Check sheet for the modelled part. Datum: model origin and axes. Units: mm. Face numbers are marked on the shaded views. A direction names the side the tool comes from. Round coordinates to 2 decimals unless told otherwise and drop trailing zeros. Loops run counter-clockwise (first coordinate to the right, second up) from the corner with the lowest first, then second, coordinate; pieces in that order, holes last. Notation, with made-up numbers: (-4, 64.25) -> (42, 64.25) arc R30 ccw to (42, 102.25) -> close; hole circle Ø5 at (-21, 32). An arc over 180 degrees is marked (long way). Use one line per item in the form item = value. Start each with the question number.
(1) Sectioned sample at C-C (y = -53). Record the cut outline in (x, z), and give its area (3 significant figures).
(2) Go/stop test with flat-tipped pins: pin 1 (2.5 mm diameter, centred on x = -0.5, y = -47.5, fed in from +Z); pin 2 (1.5 mm diameter, centred on x = 8.5, y = -50.5, fed in from -Z); pin 3 (3 mm diameter, centred on x = 11.5, y = -16.5, fed in from +Z). Record where each tip stops, or that it passes through.
(3) Material ranges on probe 1 along Y at (x, z) = (7.5, 16.25); probe 2 along X at (y, z) = (-26.5, 21); probe 3 along Y at (x, z) = (21, 14), recorded low to high. Write a range as [from, to].
(4) Sectioned sample at B-B (y = -32.5). Record the cut outline in (x, z).
(5) Draft check along X on the marked faces 5, 6, 7 and 8. Enter one of: released by +X, released by -X, zero draft, split by the parting line, or undercut.
(6) Set-up check for the marked faces 1, 2, 3 and 4: record each of +Z, -Z, +X, -X, +Y, -Y from which the full face is reachable in a straight line by a thin tool's end or side.
(7) Sectioned sample at A-A (z = 18). Record the cut outline in (x, y).
(8) Sectioned sample at D-D (z = 4.5). State how many separate pieces and enclosed holes the cut face has, and give its area (3 significant figures).
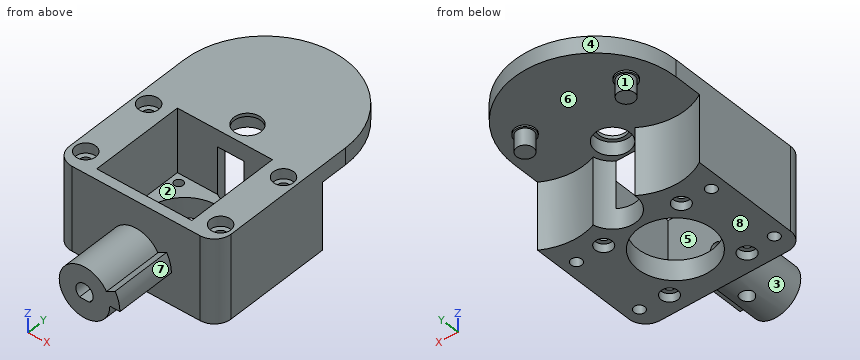
from build123d import *

# Parameters (mm, degrees)
EXTRUDE_1_DEPTH      = 25
SKETCH_3_W           = 28.2
SKETCH_3_H           = 28.2
CUT_EXTRUDE_1_DEPTH  = 19
SKETCH_4_R           = 11.1
CUT_EXTRUDE_2_DEPTH  = 26
CUT_EXTRUDE_3_DEPTH  = 20
SKETCH_11_R          = 3
EXTRUDE_2_DEPTH      = 0.5
SKETCH_12_R          = 2.5
EXTRUDE_3_DEPTH      = 5
SKETCH_13_R          = 5.05
CUT_EXTRUDE_6_DEPTH  = 4
SKETCH_14_R          = 4
CUT_EXTRUDE_7_DEPTH  = 2
SKETCH_15_R          = 1.6
CUT_EXTRUDE_8_DEPTH  = 26
SKETCH_16_R          = 3
CUT_EXTRUDE_9_DEPTH  = 3
SKETCH_17_R          = 1.3
CUT_EXTRUDE_10_DEPTH = 7
SKETCH_18_R          = 2.5
CUT_EXTRUDE_11_DEPTH = 2.5
FILLET_1_R           = 5
SKETCH_19_R          = 7.5
EXTRUDE_4_DEPTH      = 18
CUT_EXTRUDE_12_DEPTH = 18
SKETCH_21_R          = 1.5
CUT_EXTRUDE_13_DEPTH = 10
EXTRUDE_5_DEPTH      = 18
SKETCH_23_R          = 2
CUT_EXTRUDE_14_DEPTH = 8.4


with BuildPart() as part:
    # 草图1 → 凸台-拉伸1 (new body)
    with BuildSketch(Plane.XY):
        with BuildLine():
            Line((-24, 0), (-24, -45))
            Line((-24, -45), (24, -45))
            Line((24, -45), (24, 0))
            ThreePointArc((24, 0), (0, 24), (-24, 0))
        make_face()
    extrude(amount=EXTRUDE_1_DEPTH)

    # 草图3 → 切除-拉伸1 (cut)
    with BuildSketch(Plane.XY.offset(25)):
        with Locations((0, -28)):
            Rectangle(SKETCH_3_W, SKETCH_3_H)
    extrude(amount=-CUT_EXTRUDE_1_DEPTH, mode=Mode.SUBTRACT)

    # 草图4 → 切除-拉伸2 (cut, through all)
    with BuildSketch(Plane(origin=(0, 0, 0), x_dir=(-1, 0, 0), z_dir=(0, 0, -1))):
        with Locations((0, -28)):
            Circle(SKETCH_4_R)
    extrude(amount=-CUT_EXTRUDE_2_DEPTH, mode=Mode.SUBTRACT)

    # 草图8 → 切除-拉伸3 (cut)
    with BuildSketch(Plane(origin=(0, 0, 0), x_dir=(-1, 0, 0), z_dir=(0, 0, -1))):
        with BuildLine():
            Line((-24, 0), (-24, -8.109291107))
            ThreePointArc((-24, -8.109291107), (-16.458301288, -10.540093017), (-8.617628111, -9.395601202))
            ThreePointArc((-8.617628111, -9.395601202), (-0.85769165, -15.019882082), (5.242543421, -7.628246176))
            ThreePointArc((5.242543421, -7.628246176), (14.551350723, -10.595208108), (24, -8.109291107))
            Line((24, -8.109291107), (24, 0))
            ThreePointArc((24, 0), (0, 24), (-24, 0))
        make_face()
    extrude(amount=-CUT_EXTRUDE_3_DEPTH, mode=Mode.SUBTRACT)

    # 草图11 → 凸台-拉伸2 (add)
    with BuildSketch(Plane(origin=(0, 0, 20), x_dir=(-1, 0, 0), z_dir=(0, 0, -1))):
        with Locations((-15, 6.899039913)):
            Circle(SKETCH_11_R)
        with Locations((15, 6.899039913)):
            Circle(SKETCH_11_R)
    extrude(amount=EXTRUDE_2_DEPTH)

    # 草图12 → 凸台-拉伸3 (add)
    with BuildSketch(Plane(origin=(0, 0, 19.5), x_dir=(-1, 0, 0), z_dir=(0, 0, -1))):
        with Locations((-15, 6.899039913)):
            Circle(SKETCH_12_R)
        with Locations((15, 6.899039913)):
            Circle(SKETCH_12_R)
    extrude(amount=EXTRUDE_3_DEPTH)

    # 草图13 → 切除-拉伸6 (cut)
    with BuildSketch(Plane(origin=(0, 0, 20), x_dir=(-1, 0, 0), z_dir=(0, 0, -1))):
        with Locations((-1.743114855, -8.076106038)):
            Circle(SKETCH_13_R)
    extrude(amount=-CUT_EXTRUDE_6_DEPTH, mode=Mode.SUBTRACT)

    # 草图14 → 切除-拉伸7 (cut, through all)
    with BuildSketch(Plane(origin=(0, 0, 24), x_dir=(-1, 0, 0), z_dir=(0, 0, -1))):
        with Locations((-1.743114855, -8.076106038)):
            Circle(SKETCH_14_R)
    extrude(amount=-CUT_EXTRUDE_7_DEPTH, mode=Mode.SUBTRACT)

    # 草图15 → 切除-拉伸8 (cut, through all)
    with BuildSketch(Plane.XY.offset(25)):
        with Locations((-20, -39)):
            Circle(SKETCH_15_R)
        with Locations((-20, -17)):
            Circle(SKETCH_15_R)
        with Locations((20, -39)):
            Circle(SKETCH_15_R)
        with Locations((20, -17)):
            Circle(SKETCH_15_R)
    extrude(amount=-CUT_EXTRUDE_8_DEPTH, mode=Mode.SUBTRACT)

    # 草图16 → 切除-拉伸9 (cut)
    with BuildSketch(Plane.XY.offset(25)):
        with Locations((-20, -17)):
            Circle(SKETCH_16_R)
        with Locations((-20, -39)):
            Circle(SKETCH_16_R)
        with Locations((20, -17)):
            Circle(SKETCH_16_R)
        with Locations((20, -39)):
            Circle(SKETCH_16_R)
    extrude(amount=-CUT_EXTRUDE_9_DEPTH, mode=Mode.SUBTRACT)

    # 草图17 → 切除-拉伸10 (cut, through all)
    with BuildSketch(Plane.XY.offset(6)):
        with Locations((-11.5, -16.5)):
            Circle(SKETCH_17_R)
        with Locations((11.5, -16.5)):
            Circle(SKETCH_17_R)
        with Locations((11.5, -39.5)):
            Circle(SKETCH_17_R)
        with Locations((-11.5, -39.5)):
            Circle(SKETCH_17_R)
    extrude(amount=-CUT_EXTRUDE_10_DEPTH, mode=Mode.SUBTRACT)

    # 草图18 → 切除-拉伸11 (cut)
    with BuildSketch(Plane(origin=(0, 0, 0), x_dir=(-1, 0, 0), z_dir=(0, 0, -1))):
        with Locations((-11.5, -16.5)):
            Circle(SKETCH_18_R)
        with Locations((11.5, -16.5)):
            Circle(SKETCH_18_R)
        with Locations((-11.5, -39.5)):
            Circle(SKETCH_18_R)
        with Locations((11.5, -39.5)):
            Circle(SKETCH_18_R)
    extrude(amount=-CUT_EXTRUDE_11_DEPTH, mode=Mode.SUBTRACT)

    # 圆角1
    fillet_1_edges = [part.edges().sort_by_distance(p)[0] for p in [
        (24, -45, 12.5),
        (-24, -45, 12.5),
    ]]
    fillet(fillet_1_edges, radius=FILLET_1_R)

    # 草图19 → 凸台-拉伸4 (add)
    with BuildSketch(Plane.XZ.offset(45)):
        with Locations((0, 9.5)):
            Circle(SKETCH_19_R)
    extrude(amount=EXTRUDE_4_DEPTH)

    # 草图20 → 切除-拉伸12 (cut)
    with BuildSketch(Plane.XZ.offset(63)):
        with BuildLine():
            Line((-1.446547614, 7.4), (1.446547614, 7.4))
            ThreePointArc((1.446547614, 7.4), (0, 12.05), (-1.446547614, 7.4))
        make_face()
    extrude(amount=-CUT_EXTRUDE_12_DEPTH, mode=Mode.SUBTRACT)

    # 草图21 → 切除-拉伸13 (cut)
    with BuildSketch(Plane.XZ.offset(45)):
        with Locations((0, 9.5)):
            Circle(SKETCH_21_R)
    extrude(amount=-CUT_EXTRUDE_13_DEPTH, mode=Mode.SUBTRACT)

    # 草图22 → 凸台-拉伸5 (add)
    with BuildSketch(Plane.XZ.offset(45)):
        with BuildLine():
            Line((7.5, 9.5), (10.5, 9.5))
            ThreePointArc((10.5, 9.5), (10.142221176, 12.217599974), (9.09326674, 14.75))
            Line((9.09326674, 14.75), (6.495190528, 13.25))
            ThreePointArc((6.495190528, 13.25), (7.244443697, 11.441142838), (7.5, 9.5))
        make_face()
    extrude(amount=EXTRUDE_5_DEPTH)

    # 草图23 → 切除-拉伸14 (cut, through all)
    with BuildSketch(Plane.XY.offset(7.4)):
        with Locations((0, -53)):
            Circle(SKETCH_23_R)
    extrude(amount=-CUT_EXTRUDE_14_DEPTH, mode=Mode.SUBTRACT)


solid = part.part
Checks:
q1.outline = (-2, 2.27) -> (-2, 7.4) -> (-1.45, 7.4) arc R2.55 cw (long way) to (1.45, 7.4) -> (2, 7.4) -> (2, 2.27) arc R7.5 ccw to (7.5, 9.5) -> (10.5, 9.5) arc R10.5 ccw to (9.09, 14.75) -> (6.5, 13.25) arc R7.5 ccw (long way) to start
q1.area = 150 mm2
q2.pin_1 = 17
q2.pin_2 = 9.5
q2.pin_3 = 6
q3.probe_1 = [-45, -42.1], [-13.9, -12.06]
q3.probe_2 = [-24, -14.1], [14.1, 24]
q3.probe_3 = [-44.58, -40.25], [-37.75, -18.25], [-15.75, -9.54]
q4.outline = (-24, 0) -> (-10.15, 0) -> (-10.15, 6) -> (-14.1, 6) -> (-14.1, 25) -> (-24, 25) -> close; (10.15, 0) -> (24, 0) -> (24, 25) -> (14.1, 25) -> (14.1, 6) -> (10.15, 6) -> close
q5.face_5 = undercut
q5.face_6 = undercut
q5.face_7 = released by +X
q5.face_8 = zero draft
q6.face_1 = -Z
q6.face_2 = +Z
q6.face_3 = -Y
q6.face_4 = +Z, -Z, +Y
q7.outline = (-24, -40) arc R5 ccw to (-19, -45) -> (19, -45) arc R5 ccw to (24, -40) -> (24, -8.11) arc R17.5 cw to (8.62, -9.4) arc R7 cw to (5.63, -13.9) -> (14.1, -13.9) -> (14.1, -42.1) -> (-14.1, -42.1) -> (-14.1, -13.9) -> (-2.14, -13.9) arc R7 cw to (-5.24, -7.63) arc R17.5 cw to (-24, -8.11) -> close; circle Ø5 at (-15, 6.9); circle Ø5 at (15, 6.9); hole circle Ø3.2 at (-20, -39); hole circle Ø3.2 at (-20, -17); hole circle Ø3.2 at (20, -39); hole circle Ø3.2 at (20, -17)
q8.separate_pieces = 1
q8.enclosed_holes = 10
q8.area = 1,370 mm2
